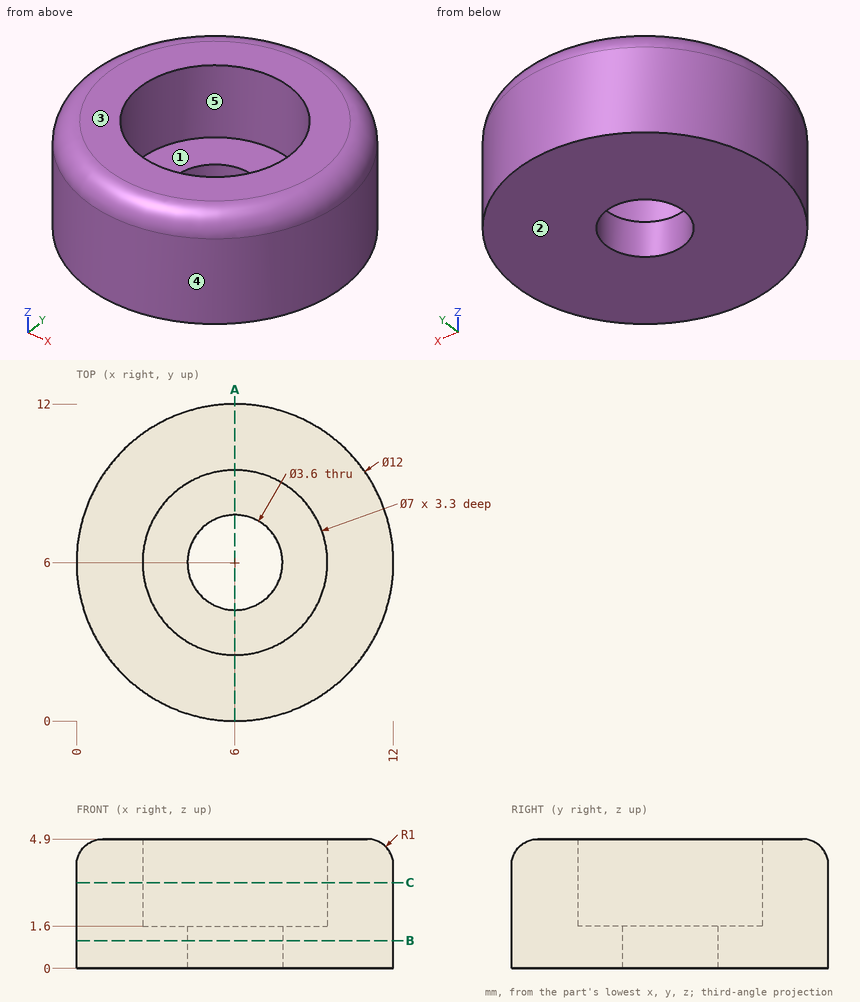
Geometry check sheet. Reference: drawing and pictorial views, mm from the part's lowest x, y, z. A direction names the side the tool comes from. Round coordinates to 2 decimals unless told otherwise and drop trailing zeros. Write each loop counter-clockwise with the first axis right and the second up, starting at its lowest first coordinate (ties: lowest second). Pieces come first, ordered by that corner, then holes.
1. Access from +Z, -Z, +X, -X, +Y, -Y to the whole of each face (thin tool, end or side, straight path). Record for the marked faces 1 and 2.
2. Section check A-A on x = 6. Enter the section's corners in (y, z), plus the area to 3 significant figures.
3. Draft check along Y on the marked faces 3, 4 and 5. Enter one of: +Y half, -Y half, draft (parallel to the pull), parting line (faces both ways), or undercut.
4. Scan lines: L1, parallel to Y at x = 6, z = 2.8; L2, parallel to X at y = 6, z = 1.05. Record each from-to range of solid material in increasing order.
5. Section check B-B on z = 1.05. Enter the section's corners in (x, y), plus the area to 3 significant figures.
6. Gauge pin test, flat ends, axial feed: P1, Ø2, axis at x = 6.5, y = 5.5, coming from the +Z side; P2, Ø1, axis at x = 7, y = 7, coming from the +Z side. Record the tip position at first contact, or that the pin passes through.
7. Section check C-C on z = 3.25. Enter the section's corners in (x, y).
Answer:
1. face 1: +Z
1. face 2: -Z, +X, -X, +Y, -Y
2. outline: (0, 0) - (4.2, 0) - (4.2, 1.6) - (2.5, 1.6) - (2.5, 4.9) - (1, 4.9) arc R1 ccw to (0, 3.9) - close; (7.8, 0) - (12, 0) - (12, 3.9) arc R1 ccw to (11, 4.9) - (9.5, 4.9) - (9.5, 1.6) - (7.8, 1.6) - close
2. area: 29.5 mm2
3. face 3: draft
3. face 4: parting line
3. face 5: undercut
4. L1: y = 0 to 2.5, 9.5 to 12
4. L2: x = 0 to 4.2, 7.8 to 12
5. outline: circle Ø12 at (6, 6); hole circle Ø3.6 at (6, 6)
5. area: 103 mm2
6. P1: passes through
6. P2: stops at z = 1.6
7. outline: circle Ø12 at (6, 6); hole circle Ø7 at (6, 6)
